Could you check a few things on this model? Use its own coordinates, in mm. A direction names the side the tool comes from. Coordinates: 2 decimals unless noted, no trailing zeros. Order: outer loops, then holes, each group sorted by start corner. A loop starts at its lowest first (then second) coordinate and runs counter-clockwise, first axis right, second up.
```python
from build123d import *

# Parameters (mm, degrees)
SKETCH1_W               = 46.5
SKETCH1_H               = 24
BOSS_EXTRUDE1_DEPTH     = 21
SHELL1_T                = -1.25
SKETCH2_W               = 19.75
SKETCH2_H               = 14.5
CUT_EXTRUDE1_DEPTH      = 57.384838388
SKETCH4_W               = 6.75
SKETCH4_H               = 6.5
SKETCH4_W_2             = 7.5
SKETCH4_H_2             = 17
CUT_EXTRUDE3_DEPTH      = 1.25
CUT_EXTRUDE4_REACH      = 57.358
SKETCH6_R               = 1.95
SKETCH7_W               = 10.375
SKETCH7_H               = 2.5
CUT_EXTRUDE5_DEPTH      = 1.25
SKETCH9_W               = 19.5
SKETCH9_H               = 6
BOSS_EXTRUDE3_DEPTH     = 2.5
CUT_EXTRUDE7_DEPTH      = 102.634838388
CUT_EXTRUDE7_DEPTH_BACK = 57.384838388
CUT_EXTRUDE7_START      = -45.25
SKETCH12_W              = 1.5
SKETCH12_H              = 8.25
SKETCH13_W              = 2.75
SKETCH13_H              = 8.25
BOSS_EXTRUDE4_DEPTH     = 44
SKETCH15_W              = 10
SKETCH15_H              = 2.75
BOSS_EXTRUDE5_DEPTH     = 0.75


with BuildPart() as part:
    # Sketch1 → Boss-Extrude1 (new body)
    with BuildSketch(Plane.XY):
        with Locations((22, 12)):
            Rectangle(SKETCH1_W, SKETCH1_H)
    extrude(amount=-BOSS_EXTRUDE1_DEPTH)

    # Shell1
    shell1_openings = [part.faces().sort_by_distance(p)[0] for p in [
        (22, 12, -21),
        (22, 24, -10.5),
    ]]
    offset(amount=SHELL1_T, openings=shell1_openings, kind=Kind.INTERSECTION)

    # Sketch2 → Cut-Extrude1 (cut, through all)
    with BuildSketch(Plane.ZY.offset(1.25)):
        with Locations((-11.125, 8.5)):
            Rectangle(SKETCH2_W, SKETCH2_H)
    extrude(amount=-CUT_EXTRUDE1_DEPTH, mode=Mode.SUBTRACT)

    # Sketch4 → Cut-Extrude3 (cut)
    with BuildSketch(Plane.XY):
        with Locations((8.375, 11.5)):
            Rectangle(SKETCH4_W, SKETCH4_H)
        with Locations((22.75, 15.75)):
            Rectangle(SKETCH4_W_2, SKETCH4_H_2)
    extrude(amount=-CUT_EXTRUDE3_DEPTH, mode=Mode.SUBTRACT)

    # Sketch6 → Cut-Extrude4 (cut, up to next)
    with BuildSketch(Plane(origin=(0, 0, 0), x_dir=(-1, 0, 0), z_dir=(0, -1, 0)), mode=Mode.PRIVATE) as cut_extrude4_sk1:
        with Locations(Location((-6.125, 9, 0), (0, 0, 90))):
            Circle(SKETCH6_R)
    cut_extrude4_tool1 = extrude(cut_extrude4_sk1.sketch, amount=-CUT_EXTRUDE4_REACH, mode=Mode.PRIVATE) & part.part
    # Sketch6 → Cut-Extrude4 (cut, up to next)
    with BuildSketch(Plane(origin=(0, 0, 0), x_dir=(-1, 0, 0), z_dir=(0, -1, 0)), mode=Mode.PRIVATE) as cut_extrude4_sk2:
        with Locations(Location((-37.875, 9, 0), (0, 0, 90))):
            Circle(SKETCH6_R)
    cut_extrude4_tool2 = extrude(cut_extrude4_sk2.sketch, amount=-CUT_EXTRUDE4_REACH, mode=Mode.PRIVATE) & part.part
    add(cut_extrude4_tool1.solids().sort_by_distance((6.125, 0, -9))[0], mode=Mode.SUBTRACT)
    add(cut_extrude4_tool2.solids().sort_by_distance((37.875, 0, -9))[0], mode=Mode.SUBTRACT)

    # Sketch7 → Cut-Extrude5 (cut)
    with BuildSketch(Plane.XY):
        with Locations((40.0625, 2.5)):
            Rectangle(SKETCH7_W, SKETCH7_H)
        with Locations((3.9375, 2.5)):
            Rectangle(SKETCH7_W, SKETCH7_H)
    extrude(amount=-CUT_EXTRUDE5_DEPTH, mode=Mode.SUBTRACT)

    # Sketch9 → Boss-Extrude3 (add)
    with BuildSketch(Plane(origin=(0, 1.25, 0), x_dir=(1, 0, 0), z_dir=(0, 1, 0))):
        with Locations((25.125, 18)):
            Rectangle(SKETCH9_W, SKETCH9_H)
    extrude(amount=BOSS_EXTRUDE3_DEPTH)

    # Sketch12 → Cut-Extrude7 (cut, two sides: drawn at the far end of the back side and taken through both)
    with BuildSketch(Plane(origin=(45.25, 0, 0), x_dir=(0, 0, -1), z_dir=(1, 0, 0)).offset(CUT_EXTRUDE7_START - CUT_EXTRUDE7_DEPTH_BACK)):
        with Locations((20.25, 19.875)):
            Rectangle(SKETCH12_W, SKETCH12_H)
    extrude(amount=CUT_EXTRUDE7_DEPTH + CUT_EXTRUDE7_DEPTH_BACK, mode=Mode.SUBTRACT)

    # Sketch13 → Boss-Extrude4 (add)
    with BuildSketch(Plane(origin=(0, 0, 0), x_dir=(0, 0, -1), z_dir=(1, 0, 0))):
        with Locations((18.125, 19.875)):
            Rectangle(SKETCH13_W, SKETCH13_H)
    extrude(amount=BOSS_EXTRUDE4_DEPTH)

    # Sketch15 → Boss-Extrude5 (add)
    with BuildSketch(Plane.XZ.offset(-15.75)):
        with Locations((29.875, -18.125)):
            Rectangle(SKETCH15_W, SKETCH15_H)
    extrude(amount=BOSS_EXTRUDE5_DEPTH)


solid = part.part
```
Item 1: Suppose I cut it at C-C (x = 32.5). List the corners of the cut face in (y, z) for me, and give its area (3 significant figures).
Item 2: Suppose I cut it at A-A (y = 12). List the corners of the cut face in (x, z) for me, and give its area (3 significant figures).
Item 3: Suppose I cut it at D-D (x = 10). List the corners of the cut face in (y, z) for me.
Item 4: Which directions (+Z, -Z, +X, -X, +Y, -Y) give clear straight access to the entire face, cutting with the end or side of a thin tool? Please do faces 4 (the face through (34.875, 2, -1)), 5 (the face through (15.375, 2, -18)), 6 (the face through (0, 20, -9)), 7 (the face through (11.75, 11, -1)), 8 (the face through (25, 2, -15)).
Item 5: Suppose I cut it at B-B (z = -19). List the corners of the cut face in (x, y) for me (3 decimals).
Item 6: Thinking about a two-plate mould opening in Y: for faces 1 (the face through (22, 1.25, -10)), 2 (the face through (23, 7.25, -1)), 3 (the face through (44, 20, -9)), which applies, +Y half, -Y half, draft (parallel to the pull), parting line (faces both ways), or undercut?
Item 7: For pin 1 Ø4 at (x, y) = (19, 17) entering from -Z; pin 2 Ø1.2 at (y, z) = (2.5, -19) entering from -X (3 decimals); pin 3 Ø1.5 at (x, y) = (16.5, 12.5) entering from -Z, each with a flat end and sliding along its axis, tell me the tip position at first contact or that it passes through.
Item 8: I need wall thicknesses on line 1 (X direction, y = 0.9, z = -9) (3 decimals); line 2 (Y direction, x = 25.5, z = -19.25); line 3 (Y direction, x = 35, z = -19.25). Which ranges of each line are inside material? Lowest first, please.
Geometry results:
1. outline: (0, -21) - (3.75, -21) - (3.75, -15) - (1.25, -15) - (1.25, -1.25) - (24, -1.25) - (24, 0) - (0, 0) - close; (15, -19.5) - (24, -19.5) - (24, -16.75) - (15, -16.75) - close
1. area: 94.4 mm2
2. outline: (-1.25, -1.25) - (5, -1.25) - (5, 0) - (-1.25, 0) - close; (11.75, -1.25) - (19, -1.25) - (19, 0) - (11.75, 0) - close; (26.5, -1.25) - (45.25, -1.25) - (45.25, 0) - (26.5, 0) - close
2. area: 40.3 mm2
3. outline: (0, -21) - (1.25, -21) - (1.25, -1.25) - (8.25, -1.25) - (8.25, 0) - (0, 0) - close; (14.75, -1.25) - (24, -1.25) - (24, 0) - (14.75, 0) - close; (15.75, -19.5) - (24, -19.5) - (24, -16.75) - (15.75, -16.75) - close
4. face 4: +Z, -Z, +X
4. face 5: -Z, -X
4. face 6: +Y
4. face 7: +Z, -Z
4. face 8: +X, -X, +Y
5. outline: (-1.25, 0) - (45.25, 0) - (45.25, 1.25) - (34.875, 1.25) - (34.875, 3.75) - (15.375, 3.75) - (15.375, 1.25) - (-1.25, 1.25) - close; (-1.25, 15.75) - (24.875, 15.75) - (24.875, 15) - (34.875, 15) - (34.875, 15.75) - (45.25, 15.75) - (45.25, 24) - (-1.25, 24) - close
6. face 1: undercut
6. face 2: +Y half
6. face 3: draft
7. pin 1: stops at z = -19.5
7. pin 2: stops at x = 15.375
7. pin 3: stops at z = -1.25
8. line 1: x = -1.25 to 4.175, 8.075 to 35.925, 39.825 to 45.25
8. line 2: y = 0 to 3.75, 15 to 24
8. line 3: y = 0 to 1.25, 15.75 to 24
